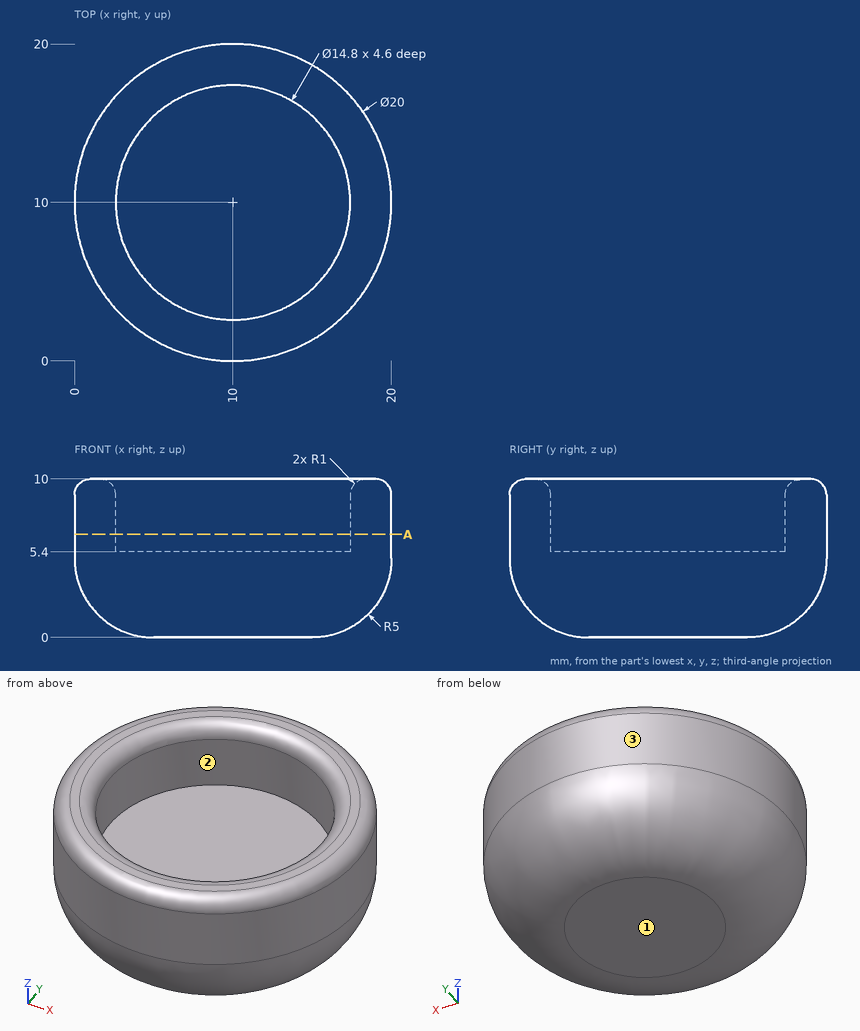
Source: three-view drawing plus pictorial views. Frame: mm from the lowest corner of the part. Give positions to 0.01 mm unless a question says otherwise; leave off trailing zeros. Order: outer loops, then holes, each group sorted by start corner. A loop starts at its lowest first (then second) coordinate and runs counter-clockwise, first axis right, second up. Notation, with made-up numbers: (9.25, 71) -> (52.25, 71) arc R18 ccw to (52.25, 79) -> close; hole circle Ø11 at (-7.5, -39.5). An arc over 180 degrees is marked (long way). Put each result on its own line as item: value.
Q1. Material intervals for L1, parallel to Y at x = 10.25, z = 7.75; L2, parallel to Z at x = 13.75, y = 12; L3, parallel to Y at x = 11.5, z = 5.5, sorted ascending.
Here are the results:
L1: y = 0 to 2.6, 17.4 to 20
L2: z = 0 to 5.4
L3: y = 0.11 to 2.75, 17.25 to 19.89
Q2. Draft query along X for the marked faces 1, 2 and 3. Return one class per face: released by +X, released by -X, zero draft, split by the parting line, or undercut.
Here are the results:
face 1: zero draft
face 2: undercut
face 3: split by the parting line
Q3. Pin query (flat end, axial travel): pin 1 (5 mm diameter, centred on y = 10, z = 1.5, fed in from -X); pin 2 (2 mm diameter, centred on x = 8, z = 7, fed in from -Y); pin 3 (1.5 mm diameter, centred on y = 14, z = 4.5, fed in from +X). Return the tip coordinate at first contact, or that it passes through.
Here are the results:
pin 1: stops at x = 0.1
pin 2: stops at y = 0.05
pin 3: stops at x = 19.44
Q4. Section A-A, the plane z = 6.5. Return loops of the section in (x, y).
Here are the results:
outline: circle Ø20 at (10, 10); hole circle Ø14.8 at (10, 10)
